Input: part model. Units: mm. Frame: model coordinates. Face numbers are marked on the shaded views. A direction names the side the tool comes from. Round coordinates to 2 decimals unless told otherwise and drop trailing zeros. Order: outer loops, then holes, each group sorted by start corner. A loop starts at its lowest first (then second) coordinate and runs counter-clockwise, first axis right, second up. Notation, with made-up numbers: M 77,-27.75 L 113,-27.75 A17 cw 113,-20.75 Z; hole C 39,-19 d11. An arc over 180 degrees is marked long. One line per question, with ' | ' between items.
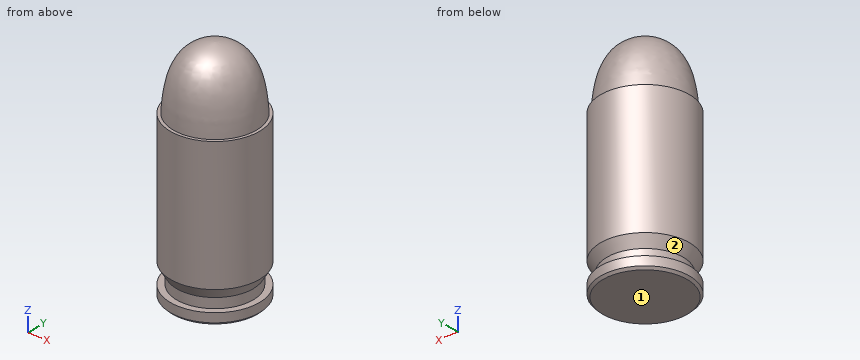
```python
from build123d import *

# Parameters (mm, degrees)
F0_W    = 4.2545
F0_H    = 1.0922
F2_SIZE = 0.254


with BuildPart() as f1:
    # F0 (on Front) → F1 (revolve)
    with BuildSketch(Plane.XZ):
        with BuildLine():
            Line((0, 14.1986), (0, 7.239))
            Line((0, 7.239), (4.6228, 7.239))
            add(Edge.make_bspline(
                [(0, 14.1986), (3.952446, 13.911695), (4.413521, 10.257011), (4.6228, 7.239)],
                knots=[0, 0, 0, 0, 8.355017, 8.355017, 8.355017, 8.355017], degree=3))
        make_face()
        Polygon((0, -7.239), (4.953, -7.239), (4.953, 7.239), (4.6228, 7.239), (0, 7.239), align=None)
        Polygon((4.2545, -8.4074), (4.953, -7.239), (0, -7.239), (0, -8.4074), align=None)
        with Locations((2.12725, -8.9535)):
            Rectangle(F0_W, F0_H)
        Polygon((4.953, -9.4996), (4.2545, -9.4996), (0, -9.4996), (0, -10.7442), (4.953, -10.7442), align=None)
    revolve(axis=Axis((0, 0, 0), (0, 0, -1)))

    # F2
    f2_edges = [f1.edges().sort_by_distance(p)[0] for p in [
        (-4.953, 0, -10.7442),
    ]]
    chamfer(f2_edges, length=F2_SIZE)


solid = f1.part
```
Item 1: Access query for the marked faces 1 and 2. Directions: +Z, -Z, +X, -X, +Y, -Y. A direction counts if a zero-diameter tool reaches every point of the face in a straight line with its end or side. Return the directions, or none.
Report:
face 1: -Z, +X, -X, +Y, -Y | face 2: none
Item 2: First-contact query: pin 1 (1 mm diameter, centred on x = 1.5, z = 3, fed in from -Y); pin 2 (5 mm diameter, centred on x = -2, y = -1, fed in from +Z); pin 3 (3 mm diameter, centred on x = -0.5, y = -2.5, fed in from +Z). Flat tips, straight axial feed; report the tip coordinate or a pass-through.
Report:
pin 1: y = -4.85 | pin 2: z = 14.2 | pin 3: z = 14.03
Item 3: Line query: line 1 along Y through (x, z) = (-0.25, 2); line 2 along Z through (x, y) = (-4, -2.5); line 3 along Z through (x, y) = (4.25, 2). Output: solid intervals per line, ascending. Write a range as from..to.
Report:
line 1: -4.95..4.95 | line 2: -10.73..-9.5, -7.63..7.24 | line 3: -10.74..-9.5, -7.67..7.24
Item 4: Section query A-A, the plane z = 4.25. Return loops of the section in (x, y).
Report:
outline: C 0,0 d9.91
